Geometry: final body of the model. Coordinates: model frame, mm. Face numbers are marked on the shaded views. A direction names the side the tool comes from. Give positions to 0.01 mm unless a question says otherwise; leave off trailing zeros. Loops run counter-clockwise (first coordinate to the right, second up) from the corner with the lowest first, then second, coordinate; pieces in that order, holes last. Notation, with made-up numbers: (74, -32) - (124, -32) arc R19 ccw to (124, -11) - close; hole circle Ø2 at (35, 5). An arc over 180 degrees is marked (long way). Use one line per item in the form item = value.
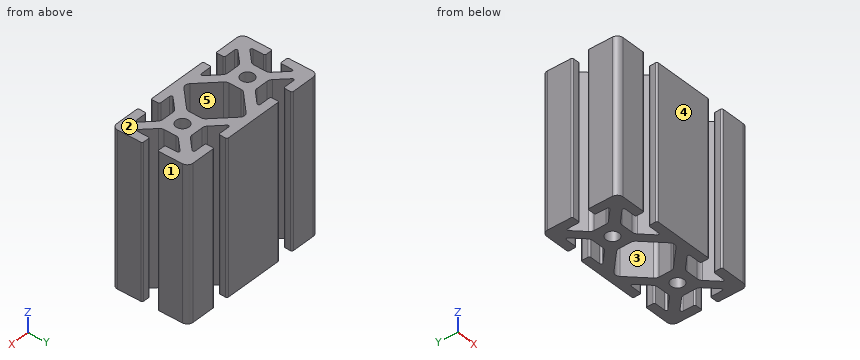
```python
from build123d import *

# Parameters (mm, degrees)
SKETCH1_R               = 3.4036
BOSS_EXTRUDE1_DEPTH     = 152.4
SKETCH2_W               = 224.8
SKETCH2_H               = 39.878
CUT_EXTRUDE1_DEPTH      = 40
CUT_EXTRUDE1_DEPTH_BACK = 40


with BuildPart() as part:
    # Sketch1 → Boss-Extrude1 (new body, symmetric)
    with BuildSketch(Plane.XY):
        with BuildLine():
            Line((-39.878, 16.891), (-39.878, 4.7625))
            ThreePointArc((-39.878, 4.7625), (-39.654815367, 4.223684633), (-39.116, 4.0005))
            Line((-39.116, 4.0005), (-36.1442, 4.0005))
            ThreePointArc((-36.1442, 4.0005), (-35.605384633, 4.223684633), (-35.3822, 4.7625))
            Line((-35.3822, 4.7625), (-35.3822, 10.2235))
            ThreePointArc((-35.3822, 10.2235), (-34.911804775, 10.927496204), (-34.081384633, 10.762315367))
            Line((-34.081384633, 10.762315367), (-28.513059555, 5.19399029))
            ThreePointArc((-28.513059555, 5.19399029), (-27.863348265, 4.221628629), (-27.6352, 3.074649845))
            Line((-27.6352, 3.074649845), (-27.6352, -3.074649845))
            ThreePointArc((-27.6352, -3.074649845), (-27.863348265, -4.221628629), (-28.513059555, -5.19399029))
            Line((-28.513059555, -5.19399029), (-34.081384633, -10.762315367))
            ThreePointArc((-34.081384633, -10.762315367), (-34.911804775, -10.927496204), (-35.3822, -10.2235))
            Line((-35.3822, -10.2235), (-35.3822, -4.7625))
            ThreePointArc((-35.3822, -4.7625), (-35.605384633, -4.223684633), (-36.1442, -4.0005))
            Line((-36.1442, -4.0005), (-39.116, -4.0005))
            ThreePointArc((-39.116, -4.0005), (-39.654815367, -4.223684633), (-39.878, -4.7625))
            Line((-39.878, -4.7625), (-39.878, -16.891))
            ThreePointArc((-39.878, -16.891), (-38.985261469, -19.046261469), (-36.83, -19.939))
            Line((-36.83, -19.939), (-24.7015, -19.939))
            ThreePointArc((-24.7015, -19.939), (-24.162684633, -19.715815367), (-23.9395, -19.177))
            Line((-23.9395, -19.177), (-23.9395, -16.2052))
            ThreePointArc((-23.9395, -16.2052), (-24.162684633, -15.666384633), (-24.7015, -15.4432))
            Line((-24.7015, -15.4432), (-30.1625, -15.4432))
            ThreePointArc((-30.1625, -15.4432), (-30.866496204, -14.972804775), (-30.701315367, -14.142384633))
            Line((-30.701315367, -14.142384633), (-25.13299029, -8.574059555))
            ThreePointArc((-25.13299029, -8.574059555), (-24.160628629, -7.924348265), (-23.013649845, -7.6962))
            Line((-23.013649845, -7.6962), (-16.864350155, -7.6962))
            ThreePointArc((-16.864350155, -7.6962), (-15.717371371, -7.924348265), (-14.74500971, -8.574059555))
            Line((-14.74500971, -8.574059555), (-9.176684633, -14.142384633))
            ThreePointArc((-9.176684633, -14.142384633), (-9.011503796, -14.972804775), (-9.7155, -15.4432))
            Line((-9.7155, -15.4432), (-15.1765, -15.4432))
            ThreePointArc((-15.1765, -15.4432), (-15.715315367, -15.666384633), (-15.9385, -16.2052))
            Line((-15.9385, -16.2052), (-15.9385, -19.177))
            ThreePointArc((-15.9385, -19.177), (-15.715315367, -19.715815367), (-15.1765, -19.939))
            Line((-15.1765, -19.939), (15.1765, -19.939))
            ThreePointArc((15.1765, -19.939), (15.715315367, -19.715815367), (15.9385, -19.177))
            Line((15.9385, -19.177), (15.9385, -16.2052))
            ThreePointArc((15.9385, -16.2052), (15.715315367, -15.666384633), (15.1765, -15.4432))
            Line((15.1765, -15.4432), (9.7155, -15.4432))
            ThreePointArc((9.7155, -15.4432), (9.011503796, -14.972804775), (9.176684633, -14.142384633))
            Line((9.176684633, -14.142384633), (14.74500971, -8.574059555))
            ThreePointArc((14.74500971, -8.574059555), (15.717371371, -7.924348265), (16.864350155, -7.6962))
            Line((16.864350155, -7.6962), (23.013649845, -7.6962))
            ThreePointArc((23.013649845, -7.6962), (24.160628629, -7.924348265), (25.13299029, -8.574059555))
            Line((25.13299029, -8.574059555), (30.701315367, -14.142384633))
            ThreePointArc((30.701315367, -14.142384633), (30.866496204, -14.972804775), (30.1625, -15.4432))
            Line((30.1625, -15.4432), (24.7015, -15.4432))
            ThreePointArc((24.7015, -15.4432), (24.162684633, -15.666384633), (23.9395, -16.2052))
            Line((23.9395, -16.2052), (23.9395, -19.177))
            ThreePointArc((23.9395, -19.177), (24.162684633, -19.715815367), (24.7015, -19.939))
            Line((24.7015, -19.939), (36.83, -19.939))
            ThreePointArc((36.83, -19.939), (38.985261469, -19.046261469), (39.878, -16.891))
            Line((39.878, -16.891), (39.878, -4.7625))
            ThreePointArc((39.878, -4.7625), (39.654815367, -4.223684633), (39.116, -4.0005))
            Line((39.116, -4.0005), (36.1442, -4.0005))
            ThreePointArc((36.1442, -4.0005), (35.605384633, -4.223684633), (35.3822, -4.7625))
            Line((35.3822, -4.7625), (35.3822, -10.2235))
            ThreePointArc((35.3822, -10.2235), (34.911804775, -10.927496204), (34.081384633, -10.762315367))
            Line((34.081384633, -10.762315367), (28.513059555, -5.19399029))
            ThreePointArc((28.513059555, -5.19399029), (27.863348265, -4.221628629), (27.6352, -3.074649845))
            Line((27.6352, -3.074649845), (27.6352, 3.074649845))
            ThreePointArc((27.6352, 3.074649845), (27.863348265, 4.221628629), (28.513059555, 5.19399029))
            Line((28.513059555, 5.19399029), (34.081384633, 10.762315367))
            ThreePointArc((34.081384633, 10.762315367), (34.911804775, 10.927496204), (35.3822, 10.2235))
            Line((35.3822, 10.2235), (35.3822, 4.7625))
            ThreePointArc((35.3822, 4.7625), (35.605384633, 4.223684633), (36.1442, 4.0005))
            Line((36.1442, 4.0005), (39.116, 4.0005))
            ThreePointArc((39.116, 4.0005), (39.654815367, 4.223684633), (39.878, 4.7625))
            Line((39.878, 4.7625), (39.878, 16.891))
            ThreePointArc((39.878, 16.891), (38.985261469, 19.046261469), (36.83, 19.939))
            Line((36.83, 19.939), (24.7015, 19.939))
            ThreePointArc((24.7015, 19.939), (24.162684633, 19.715815367), (23.9395, 19.177))
            Line((23.9395, 19.177), (23.9395, 16.2052))
            ThreePointArc((23.9395, 16.2052), (24.162684633, 15.666384633), (24.7015, 15.4432))
            Line((24.7015, 15.4432), (30.1625, 15.4432))
            ThreePointArc((30.1625, 15.4432), (30.866496204, 14.972804775), (30.701315367, 14.142384633))
            Line((30.701315367, 14.142384633), (25.13299029, 8.574059555))
            ThreePointArc((25.13299029, 8.574059555), (24.160628629, 7.924348265), (23.013649845, 7.6962))
            Line((23.013649845, 7.6962), (16.864350155, 7.6962))
            ThreePointArc((16.864350155, 7.6962), (15.717371371, 7.924348265), (14.74500971, 8.574059555))
            Line((14.74500971, 8.574059555), (9.176684633, 14.142384633))
            ThreePointArc((9.176684633, 14.142384633), (9.011503796, 14.972804775), (9.7155, 15.4432))
            Line((9.7155, 15.4432), (15.1765, 15.4432))
            ThreePointArc((15.1765, 15.4432), (15.715315367, 15.666384633), (15.9385, 16.2052))
            Line((15.9385, 16.2052), (15.9385, 19.177))
            ThreePointArc((15.9385, 19.177), (15.715315367, 19.715815367), (15.1765, 19.939))
            Line((15.1765, 19.939), (-15.1765, 19.939))
            ThreePointArc((-15.1765, 19.939), (-15.715315367, 19.715815367), (-15.9385, 19.177))
            Line((-15.9385, 19.177), (-15.9385, 16.2052))
            ThreePointArc((-15.9385, 16.2052), (-15.715315367, 15.666384633), (-15.1765, 15.4432))
            Line((-15.1765, 15.4432), (-9.7155, 15.4432))
            ThreePointArc((-9.7155, 15.4432), (-9.011503796, 14.972804775), (-9.176684633, 14.142384633))
            Line((-9.176684633, 14.142384633), (-14.74500971, 8.574059555))
            ThreePointArc((-14.74500971, 8.574059555), (-15.717371371, 7.924348265), (-16.864350155, 7.6962))
            Line((-16.864350155, 7.6962), (-23.013649845, 7.6962))
            ThreePointArc((-23.013649845, 7.6962), (-24.160628629, 7.924348265), (-25.13299029, 8.574059555))
            Line((-25.13299029, 8.574059555), (-30.701315367, 14.142384633))
            ThreePointArc((-30.701315367, 14.142384633), (-30.866496204, 14.972804775), (-30.1625, 15.4432))
            Line((-30.1625, 15.4432), (-24.7015, 15.4432))
            ThreePointArc((-24.7015, 15.4432), (-24.162684633, 15.666384633), (-23.9395, 16.2052))
            Line((-23.9395, 16.2052), (-23.9395, 19.177))
            ThreePointArc((-23.9395, 19.177), (-24.162684633, 19.715815367), (-24.7015, 19.939))
            Line((-24.7015, 19.939), (-36.83, 19.939))
            ThreePointArc((-36.83, 19.939), (-38.985261469, 19.046261469), (-39.878, 16.891))
        make_face()
        with Locations((-19.939, 0)):
            Circle(SKETCH1_R, mode=Mode.SUBTRACT)
        with Locations((19.939, 0)):
            Circle(SKETCH1_R, mode=Mode.SUBTRACT)
        with BuildLine():
            Line((-12.2428, 3.074649845), (-12.2428, -3.074649845))
            ThreePointArc((-12.2428, -3.074649845), (-12.014651735, -4.221628629), (-11.364940445, -5.19399029))
            Line((-11.364940445, -5.19399029), (-1.904671503, -14.654259232))
            ThreePointArc((-1.904671503, -14.654259232), (0, -15.4432), (1.904671503, -14.654259232))
            Line((1.904671503, -14.654259232), (11.364940445, -5.19399029))
            ThreePointArc((11.364940445, -5.19399029), (12.014651735, -4.221628629), (12.2428, -3.074649845))
            Line((12.2428, -3.074649845), (12.2428, 3.074649845))
            ThreePointArc((12.2428, 3.074649845), (12.014651735, 4.221628629), (11.364940445, 5.19399029))
            Line((11.364940445, 5.19399029), (1.904671503, 14.654259232))
            ThreePointArc((1.904671503, 14.654259232), (0, 15.4432), (-1.904671503, 14.654259232))
            Line((-1.904671503, 14.654259232), (-11.364940445, 5.19399029))
            ThreePointArc((-11.364940445, 5.19399029), (-12.014651735, 4.221628629), (-12.2428, 3.074649845))
        make_face(mode=Mode.SUBTRACT)
    extrude(amount=BOSS_EXTRUDE1_DEPTH, both=True)

    # Sketch2 → Cut-Extrude1 (cut, two sides)
    with BuildSketch(Plane(origin=(0, 0, 0), x_dir=(0, 0, -1), z_dir=(1, 0, 0))) as cut_extrude1_sk:
        with Locations((40, 0)):
            Rectangle(SKETCH2_W, SKETCH2_H)
    extrude(amount=CUT_EXTRUDE1_DEPTH, mode=Mode.SUBTRACT)
    extrude(cut_extrude1_sk.sketch, amount=-CUT_EXTRUDE1_DEPTH_BACK, mode=Mode.SUBTRACT)


solid = part.part
```
(1) Pull-direction query (X, two-part tool) for the marked faces 1, 2 and 3; classes: released by +X, released by -X, zero draft, split by the parting line, or undercut.
Solution:
face_1 = released by +X
face_2 = zero draft
face_3 = undercut
(2) Pin query (flat end, axial travel): P1, Ø2.5, axis at x = -37.5, z = 115, coming from the +Y side; P2, Ø1.8, axis at x = -20.5, z = 107.5, coming from the -Y side; P3, Ø1.5, axis at x = -38, z = 126.5, coming from the -Y side. Return the tip coordinate at first contact, or that it passes through.
Solution:
P1 = 19.94
P2 = -7.7
P3 = -19.91
(3) Cut plane A-A (y = 0). Return the cut outline in (x, z).
Solution:
outline = (-27.64, 72.4) - (-23.34, 72.4) - (-23.34, 152.4) - (-27.64, 152.4) - close; (-16.54, 72.4) - (-12.24, 72.4) - (-12.24, 152.4) - (-16.54, 152.4) - close; (12.24, 72.4) - (16.54, 72.4) - (16.54, 152.4) - (12.24, 152.4) - close; (23.34, 72.4) - (27.64, 72.4) - (27.64, 152.4) - (23.34, 152.4) - close
(4) Access query for the marked faces 4 and 5. Directions: +Z, -Z, +X, -X, +Y, -Y. A direction counts if a zero-diameter tool reaches every point of the face in a straight line with its end or side. Return the directions, or none.
Solution:
face_4 = +Z, -Z, +X, -X, -Y
face_5 = +Z, -Z
(5) Cut plane B-B (z = 122.5). Give the number of separate pieces and of enclosed holes in the cut face, plus the area to 3 significant figures.
Solution:
separate_pieces = 1
enclosed_holes = 3
area = 1,620 mm2
(6) Material intervals for L1, parallel to X at y = -17, z = 140.5; L2, parallel to X at y = 0, z = 113; L3, parallel to Y at x = 12.5, z = 140.5, sorted ascending. Write a range as from..to.
Solution:
L1 = -39.88..-23.94, -15.94..15.94, 23.94..39.88
L2 = -27.64..-23.34, -16.54..-12.24, 12.24..16.54, 23.34..27.64
L3 = -19.94..-15.44, -10.82..10.82, 15.44..19.94
(7) Cut plane C-C (y = 13). Return the cut outline in (x, z).
Solution:
outline = (-39.88, 72.4) - (-29.56, 72.4) - (-29.56, 152.4) - (-39.88, 152.4) - close; (-10.32, 72.4) - (-3.56, 72.4) - (-3.56, 152.4) - (-10.32, 152.4) - close; (3.56, 72.4) - (10.32, 72.4) - (10.32, 152.4) - (3.56, 152.4) - close; (29.56, 72.4) - (39.88, 72.4) - (39.88, 152.4) - (29.56, 152.4) - close
